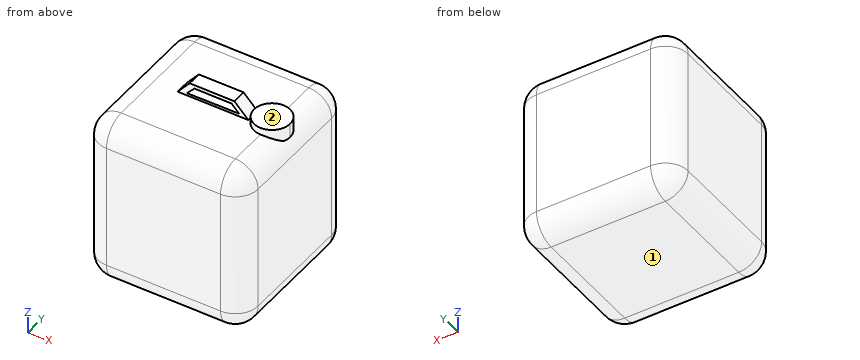
```python
from build123d import *

# Parameters (mm, degrees)
F1_DEPTH = 300
F2_R     = 40
F4_DEPTH = 12.5
F6_DEPTH = 12.5


with BuildPart() as f1:
    # F0 (on Top) → F1 (new body)
    with BuildSketch(Plane.XY):
        with BuildLine():
            ThreePointArc((140, 100), (128.2842712475, 128.2842712475), (100, 140))
            Line((100, 140), (-100, 140))
            ThreePointArc((-100, 140), (-128.2842712475, 128.2842712475), (-140, 100))
            Line((-140, 100), (-140, -100))
            ThreePointArc((-140, -100), (-128.2842712475, -128.2842712475), (-100, -140))
            Line((-100, -140), (100, -140))
            ThreePointArc((100, -140), (128.2842712475, -128.2842712475), (140, -100))
            Line((140, -100), (140, 100))
        make_face()
    extrude(amount=F1_DEPTH)

    # F2
    f2_edges = [f1.edges().sort_by_distance(p)[0] for p in [
        (128.284271, 128.284271, 300),
        (0, 140, 300),
        (-128.284271, 128.284271, 300),
        (-140, 0, 300),
        (-128.284271, -128.284271, 300),
        (0, -140, 300),
        (128.284271, -128.284271, 300),
        (140, 0, 300),
        (140, 0, 0),
    ]]
    fillet(f2_edges, radius=F2_R)

    # F3 (on face) → F4 (join, symmetric)
    with BuildSketch(Plane.XY.offset(300)):
        with BuildLine():
            ThreePointArc((100, -31.6815127242), (122.4022124856, -22.4022124855), (131.6815127242, 0))
            ThreePointArc((131.6815127242, 0), (122.4022124856, 22.4022124855), (100, 31.6815127242))
            Line((100, 31.6815127242), (100, -31.6815127242))
        make_face()
        with BuildLine():
            Line((100, -31.6815127242), (100, 31.6815127242))
            ThreePointArc((100, 31.6815127242), (68.3184872758, 0), (100, -31.6815127242))
        make_face()
    extrude(amount=F4_DEPTH, both=True)

    # F5 (on Front) → F6 (join, symmetric)
    with BuildSketch(Plane.XZ):
        Polygon((-36.387193948, 324.7865736485), (-57.6208606362, 299.7408509254), (66.6310936213, 299.7408509254), (42.0579239726, 324.7865736485), align=None)
        Polygon((50.280045718, 304.940700531), (-40.9793257713, 304.2699992657), (-28.1326603144, 318.3833062649), (37.1089726686, 318.3833062649), align=None, mode=Mode.SUBTRACT)
    extrude(amount=F6_DEPTH, both=True)


solid = f1.part
```
Geometry: final body of the model. Coordinates: model frame, mm. Face numbers are marked on the shaded views. A direction names the side the tool comes from. Give positions to 0.01 mm unless a question says otherwise; leave off trailing zeros. Loops run counter-clockwise (first coordinate to the right, second up) from the corner with the lowest first, then second, coordinate; pieces in that order, holes last. Notation, with made-up numbers: (-27, -27.5) -> (-8, -27.5) arc R5 ccw to (-8, -22.5) -> close; hole circle Ø3 at (64.25, 69). An arc over 180 degrees is marked (long way). Use CSV: the item, a comma, the result in double quotes.
(1) First-contact query: P1, Ø2, axis at x = 131, y = 2, coming from the -Z side; P2, Ø3, axis at x = -37, y = -34.5, coming from the +Z side. Flat tips, straight axial feed; report the tip coordinate or a pass-through.
From the geometry:
P1,"z = 13.54"
P2,"z = 300"
(2) Access query for the marked faces 1 and 2. Directions: +Z, -Z, +X, -X, +Y, -Y. A direction counts if a zero-diameter tool reaches every point of the face in a straight line with its end or side. Return the directions, or none.
From the geometry:
face 1,"-Z, +X, -X, +Y, -Y"
face 2,"+Z, +X, +Y, -Y"
(3) Cut plane A-A (z = 152). Output: boundary loops of the cut face in (x, y).
From the geometry:
outline,"(-140, -100) arc R40 ccw to (-100, -140) -> (100, -140) arc R40 ccw to (140, -100) -> (140, 100) arc R40 ccw to (100, 140) -> (-100, 140) arc R40 ccw to (-140, 100) -> close"
(4) Ray query, line 1 along Y through (x, z) = (84, 262.5); line 2 along Z through (x, y) = (-21, 52.5); line 3 along Y through (x, z) = (100.5, 254). Return the intervals inside material, ascending. Write a range as [from, to].
From the geometry:
line 1,"[-139.92, 139.92]"
line 2,"[0, 300]"
line 3,"[-140, 140]"
(5) Cut plane B-B (y = 55.5). Output: boundary loops of the cut face in (x, z), plus the area to 3 significant figures.
From the geometry:
outline,"(-140, 40) arc R40 ccw to (-100, 0) -> (100, 0) arc R40 ccw to (140, 40) -> (140, 260) arc R40 ccw to (100, 300) -> (-100, 300) arc R40 ccw to (-140, 260) -> close"
area,"82,600 mm^2"
(6) Cut plane C-C (x = 75.5). Output: boundary loops of the cut face in (y, z).
From the geometry:
outline,"(-140, 40) arc R40 ccw to (-100, 0) -> (100, 0) arc R40 ccw to (140, 40) -> (140, 260) arc R40 ccw to (100, 300) -> (20.09, 300) -> (20.09, 312.5) -> (-20.09, 312.5) -> (-20.09, 300) -> (-100, 300) arc R40 ccw to (-140, 260) -> close"
